Geometry check sheet. Reference: the model listing, model coordinates, mm. Face numbers are marked on the shaded views. A direction names the side the tool comes from. Coordinates: 2 decimals unless noted, no trailing zeros. Order: outer loops, then holes, each group sorted by start corner. A loop starts at its lowest first (then second) coordinate and runs counter-clockwise, first axis right, second up. Notation, with made-up numbers: M 18,72 L 29,72 A21 cw 29,87 Z; hole C 22.25,-27.75 d7. An arc over 180 degrees is marked long. Use CSV: the item, a comma, the result in double quotes. Start each with the question number.
```python
from build123d import *

# Parameters (mm, degrees)
BOSS_EXTRUDE1_DEPTH = 3.85
CHAMFER1_SIZE       = 1


with BuildPart() as part:
    # Sketch1 → Boss-Extrude1 (new body)
    with BuildSketch(Plane(origin=(0, 0, 0), x_dir=(1, 0, 0), z_dir=(0, 1, 0))):
        with BuildLine():
            Line((0, 50), (0, 47.35))
            Line((0, 47.35), (5, 47.35))
            Line((5, 47.35), (5, 43.5))
            Line((5, 43.5), (0, 43.5))
            Line((0, 43.5), (0, 40))
            ThreePointArc((0, 40), (28.284271247, 28.284271247), (40, 0))
            Line((40, 0), (42.65, 0))
            Line((42.65, 0), (42.65, 5))
            Line((42.65, 5), (46.5, 5))
            Line((46.5, 5), (46.5, 0))
            Line((46.5, 0), (50, 0))
            ThreePointArc((50, 0), (35.355339059, 35.355339059), (0, 50))
        make_face()
    extrude(amount=BOSS_EXTRUDE1_DEPTH)

    # Chamfer1
    chamfer1_edges = [part.edges().sort_by_distance(p)[0] for p in [
        (0, 1.925, -43.5),
        (0, 1.925, -47.35),
        (46.5, 1.925, 0),
        (42.65, 1.925, 0),
    ]]
    chamfer(chamfer1_edges, length=CHAMFER1_SIZE)


solid = part.part
```
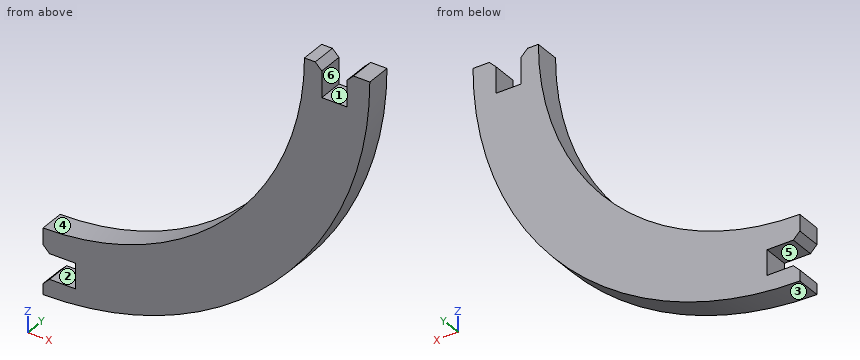
1) Section check A-A on y = 3.1. Record the boundary of the cut face in (x, z), then the cut area to 3 significant figures.
2) Material ranges on line 1 along Z through (x, y) = (3, 1.5); line 2 along X through (y, z) = (0.8, -45.5); line 3 along Z through (x, y) = (13, 2.2), recorded low to high.
3) Section check C-C on z = -45. Record the boundary of the cut face in (x, y).
4) Set-up check for the marked faces 4, 5 and 6: record each of +Z, -Z, +X, -X, +Y, -Y from which the full face is reachable in a straight line by a thin tool's end or side.
5) Gauge pin test, flat ends, axial feed: P1, Ø1.2, axis at x = 3.5, y = 2, coming from the -Z side; P2, Ø1.5, axis at x = 6, y = 1.5, coming from the -Z side; P3, Ø1.9, axis at y = 2.5, z = -2.5, coming from the +X side; P4, Ø2, axis at x = 40, z = -33, coming from the +Y side. Record the tip position at first contact, or that the pin passes through.
6) Draft check along X on the marked faces 1, 2 and 3. Enter one of: +X half, -X half, draft (parallel to the pull), parting line (faces both ways), or undercut.
7) Section check B-B on x = 23. Record the boundary of the cut face in (y, z).
Results are:
1,outline,"M 0,-50 A50 ccw 50,0 L 47.5,0 L 46.5,-1 L 46.5,-5 L 42.65,-5 L 42.65,-1 L 41.65,0 L 40,0 A40 cw 0,-40 L 0,-42.5 L 1,-43.5 L 5,-43.5 L 5,-47.35 L 1,-47.35 L 0,-48.35 Z"
1,area,"666 mm²"
2,line 1,"z = -49.91 to -47.35, -43.5 to -39.89"
2,line 2,"x = 5 to 20.73"
2,line 3,"z = -48.28 to -37.83"
3,outline,"M 5,0 L 21.79,0 L 21.79,3.85 L 5,3.85 Z"
4,face 4,"+Z, -X, +Y, -Y"
4,face 5,"-X, +Y, -Y"
4,face 6,"+Z, +Y, -Y"
5,P1,"stops at z = -49.92"
5,P2,"stops at z = -49.72"
5,P3,"stops at x = 49.98"
5,P4,"passes through"
6,face 1,"undercut"
6,face 2,"draft"
6,face 3,"+X half"
7,outline,"M 0,-44.4 L 3.85,-44.4 L 3.85,-32.73 L 0,-32.73 Z"
